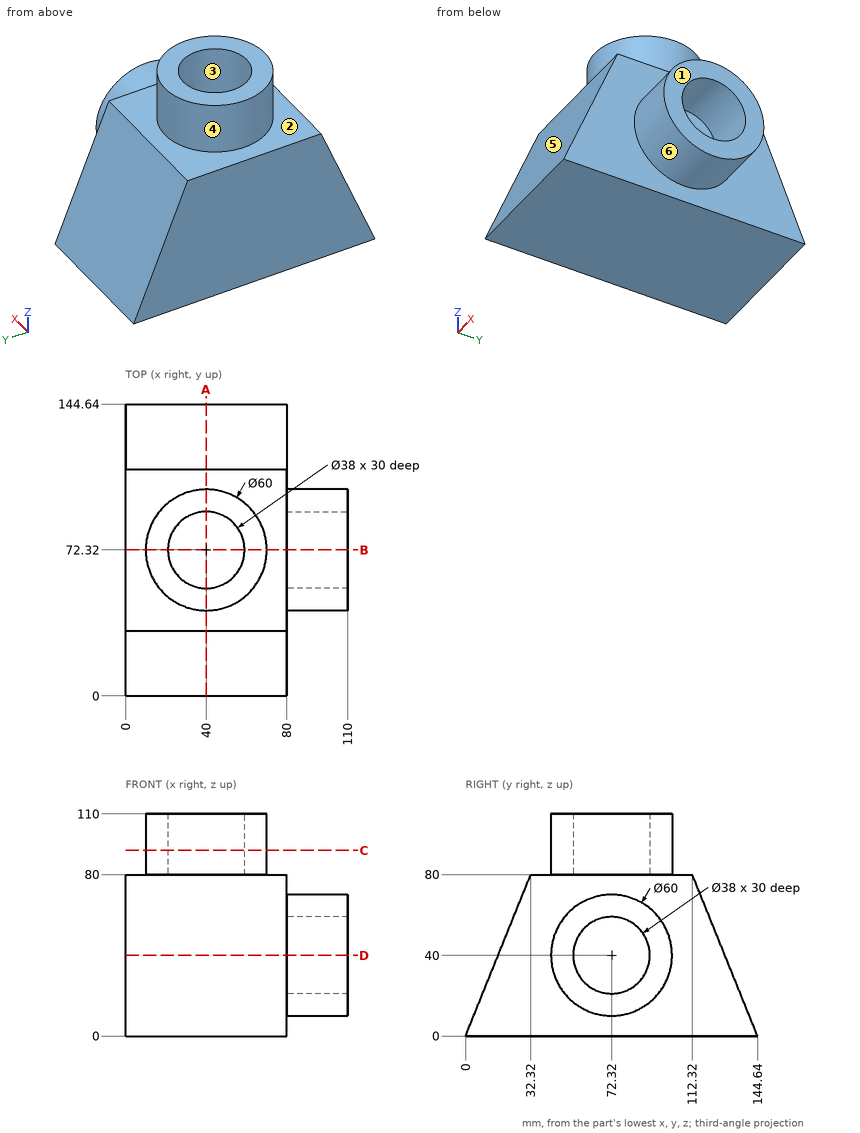
Design review of the part shown in the three views and the two pictorial views. Dimensions are in mm from the part's minimum x, y and z. A direction names the side the tool comes from. Round coordinates to 2 decimals unless told otherwise and drop trailing zeros. Write each loop counter-clockwise with the first axis right and the second up, starting at its lowest first coordinate (ties: lowest second). Pieces come first, ordered by that corner, then holes. Notation, with made-up numbers: M 14.25,31.25 L 22.25,31.25 A15 ccw 22.25,38.25 Z; hole C -13,57 d10. An arc over 180 degrees is marked long. Use a Markdown table: item, result. Add a question column.
Q1. Insertion check: pin 1 (2 mm diameter, centred on x = 39, z = 97, fed in from -Y); pin 2 (1 mm diameter, centred on y = 114.5, z = 30, fed in from +X); pin 3 (8 mm diameter, centred on x = 51, z = 60.5, fed in from -Y). Each pin has a flat end and moves straight along its axis. Give the tip position at first contact, or say it passes through.
Q2. We need section D-D, the plane z = 40. State the section outline as (x, y) points, plus the area to 3 significant figures.
Q3. We need section C-C, the plane z = 92. State the section outline as (x, y) points, plus the area to 3 significant figures.
Q4. Machinability: for the marked faces 5 and 6, which of the approach directions +Z, -Z, +X, -X, +Y, -Y give a long, thin tool a straight path to every point of the face, cutting with its end or side? Answer none if there is none.
Q5. We need section B-B, the plane y = 72.32. State the section outline as (x, z) points, plus the area to 3 significant figures.
Q6. To check wall thickness, follow line 1 (X direction, y = 72, z = 103); line 2 (Y direction, x = 40, z = 96.5). State the ranges of each line that lie inside material, in increasing order.
Q7. The part is to be moulded in two halves that separate along X. For the marked faces 1, 2, 3 and 4, say which applies: pulls with the +X half, pulls with the -X half, needs draft (parallel to the pull), parting line crosses it, or undercut.
Q8. We need section A-A, the plane x = 40. State the section outline as (y, z) points.
Findings below:
| question | item | result |
|---|---|---|
| 1 | pin 1 | stops at y = 42.32 |
| 1 | pin 2 | stops at x = 80 |
| 1 | pin 3 | stops at y = 22.83 |
| 2 | outline | M 0,16.16 L 80,16.16 L 80,42.32 L 110,42.32 L 110,53.32 L 80,53.32 L 80,91.32 L 110,91.32 L 110,102.32 L 80,102.32 L 80,128.48 L 0,128.48 Z |
| 2 | area | 9,650 mm² |
| 3 | outline | C 40,72.32 d60; hole C 40,72.32 d38 |
| 3 | area | 1,690 mm² |
| 4 | face 5 | +Z, +X, -X, -Y |
| 4 | face 6 | +X |
| 5 | outline | M 0,0 L 80,0 L 80,10 L 110,10 L 110,21 L 80,21 L 80,59 L 110,59 L 110,70 L 80,70 L 80,80 L 70,80 L 70,110 L 59,110 L 59,80 L 21,80 L 21,110 L 10,110 L 10,80 L 0,80 Z |
| 5 | area | 7,720 mm² |
| 6 | line 1 | x = 10 to 21, 59 to 70 |
| 6 | line 2 | y = 42.32 to 53.32, 91.32 to 102.32 |
| 7 | face 1 | pulls with the +X half |
| 7 | face 2 | needs draft |
| 7 | face 3 | undercut |
| 7 | face 4 | parting line crosses it |
| 8 | outline | M 0,0 L 144.64,0 L 112.32,80 L 102.32,80 L 102.32,110 L 91.32,110 L 91.32,80 L 53.32,80 L 53.32,110 L 42.32,110 L 42.32,80 L 32.32,80 Z |
